from build123d import *

# Parameters (mm, degrees)
F2_R    = 1
F3_R    = 0.5
F4_SIZE = 1


with BuildPart() as f1:
    # F0 (on Top) → F1 (revolve)
    with BuildSketch(Plane.XY):
        Polygon((1.9, 10.791767), (1.9, 5.2), (4.3, 4), (4.3, 0), (8, 0), (8, 8), (7, 9), (8, 10), (8, 13), (7, 14), (8, 15), (8, 17), (0, 17), (0, 10.791767), align=None)
    revolve(axis=Axis((0, 8.531952, 0), (0, 1, 0)))

    # F2
    f2_edges = [f1.edges().sort_by_distance(p)[0] for p in [
        (-4.3, 4, 0),
    ]]
    fillet(f2_edges, radius=F2_R)

    # F3
    f3_edges = [f1.edges().sort_by_distance(p)[0] for p in [
        (-8, 17, 0),
    ]]
    fillet(f3_edges, radius=F3_R)

    # F4
    f4_edges = [f1.edges().sort_by_distance(p)[0] for p in [
        (-8, 0, 0),
    ]]
    chamfer(f4_edges, length=F4_SIZE)


solid = f1.part
The model under review builds one solid part; all positions refer to its coordinate system, in mm. A direction names the side the tool comes from. Round coordinates to 2 decimals unless told otherwise and drop trailing zeros. Loops run counter-clockwise (first coordinate to the right, second up) from the corner with the lowest first, then second, coordinate; pieces in that order, holes last. Notation, with made-up numbers: M 38.25,-29.5 L 55.25,-29.5 A29 cw 55.25,2.5 Z; hole C 63,39.25 d8. An arc over 180 degrees is marked long. Answer as CSV lines item,"result". Start each with the question number.
Item 1: Consider section D-D (y = 15.75). Write out the cut boundary in (x, z), then the cut area to 3 significant figures.
Item 2: Consider section A-A (y = 9.75). Write out the cut boundary in (x, z), then the cut area to 3 significant figures.
Item 3: Wall thickness on line 1 (Y direction, x = 7, z = 1.75); line 2 (Z direction, x = 0, y = 1.55); line 3 (X direction, y = 6.4, z = 0): over which ranges is each line inside the solid? List them lowest first. Write a range as [from, to].
Item 4: For faces 1 (the face through (-1.73, 11.52, 7.81)), 2 (the face through (0, 10.792, 0)), list the 3-axis set-ups (+Z, -Z, +X, -X, +Y, -Y) from which the entire face can be reached by the end or side of a thin tool; tool diameter is ignored.
Item 5: Consider section C-C (z = 7.25). State how many separate pieces and enclosed holes the cut face has, then the cut area to 3 significant figures.
Item 6: Consider section B-B (y = 13.25). Write out the cut boundary in (x, z).
Item 7: Insertion check: P1, Ø4, axis at x = 0.5, z = 0, coming from the -Y side. The pin has a flat end and moves straight along its axis. Give the tip position at first contact, or say it passes through.
Item 8: Mouldability with a two-part tool opening along Z and no side actions: class faces 3 (the face through (0, 17, 0)), 4 (the face through (-1.73, 4.55, 7.81)), 5 (the face through (-1.9, 7.96, -0.08)) as released by +Z, released by -Z, zero draft, split by the parting line, or undercut.
Answer:
1,outline,"C 0,0 d16"
1,area,"201 mm^2"
2,outline,"C 0,0 d15.5; hole C 0,0 d3.8"
2,area,"177 mm^2"
3,line 1,"y = [0.22, 8.78], [9.22, 13.78], [14.22, 17]"
3,line 2,"z = [-8, -4.3], [4.3, 8]"
3,line 3,"x = [-8, -1.9], [1.9, 8]"
4,face 1,"+Y, -Y"
4,face 2,"-Y"
5,separate pieces,"3"
5,enclosed holes,"0"
5,area,"97.6 mm^2"
6,outline,"C 0,0 d15.5"
7,P1,"stops at y = 4.9"
8,face 3,"zero draft"
8,face 4,"split by the parting line"
8,face 5,"undercut"
